Verification items for the finished model (mm, model axes). A direction names the side the tool comes from. Coordinates: 2 decimals unless noted, no trailing zeros. Write each loop counter-clockwise with the first axis right and the second up, starting at its lowest first coordinate (ties: lowest second). Pieces come first, ordered by that corner, then holes. Notation, with made-up numbers: M 18,44 L 56,44 A21 cw 56,83 Z; hole C 34,1.25 d5. An arc over 180 degrees is marked long. One line per item, written item: value.
```python
from build123d import *

# Parameters (mm, degrees)
SKETCH2_W           = 220
SKETCH2_H           = 140
BOSS_EXTRUDE1_DEPTH = 2
CUT_EXTRUDE1_DEPTH  = 2
SKETCH4_W           = 8
SKETCH4_H           = 20
BOSS_EXTRUDE2_DEPTH = 2
SKETCH5_W           = 4
SKETCH5_H           = 4.381248614
BOSS_EXTRUDE3_DEPTH = 20


with BuildPart() as part:
    # Sketch2 → Boss-Extrude1 (new body)
    with BuildSketch(Plane(origin=(0, 0, 0), x_dir=(1, 0, 0), z_dir=(0, 1, 0))):
        Rectangle(SKETCH2_W, SKETCH2_H)
    extrude(amount=BOSS_EXTRUDE1_DEPTH)

    # Sketch3 → Cut-Extrude1 (cut)
    with BuildSketch(Plane(origin=(0, 0, 0), x_dir=(1, 0, 0), z_dir=(0, 1, 0))):
        Polygon((-80, -35), (-80, -22), (-85, -22), (-85, -68), (-80, -68), (-80, -55), (80, -55), (80, -68), (85, -68), (85, -22), (80, -22), (80, -35), align=None)
    extrude(amount=CUT_EXTRUDE1_DEPTH, mode=Mode.SUBTRACT)

    # Sketch4 → Boss-Extrude2 (add)
    with BuildSketch(Plane(origin=(0, 0, 0), x_dir=(1, 0, 0), z_dir=(0, 1, 0))):
        with Locations((0, -45)):
            Rectangle(SKETCH4_W, SKETCH4_H)
    extrude(amount=BOSS_EXTRUDE2_DEPTH)

    # Sketch5 → Boss-Extrude3 (add)
    with BuildSketch(Plane(origin=(0, 2, 0), x_dir=(1, 0, 0), z_dir=(0, 1, 0))):
        with Locations((-2, -42.809375693)):
            Rectangle(SKETCH5_W, SKETCH5_H)
    extrude(amount=BOSS_EXTRUDE3_DEPTH)


solid = part.part
```
Item 1: Cross-section at C-C, the plane y = 15.5. Enter the section's corners in (x, z).
The answers:
outline: M -4,40.62 L 0,40.62 L 0,45 L -4,45 Z
Item 2: Go/stop test with flat-tipped pins: P1, Ø10, axis at x = -72, y = 6.5, coming from the -Z side; P2, Ø10, axis at x = 34.5, z = 46, coming from the -Y side; P3, Ø1.2, axis at x = -1, y = 9, coming from the -Z side; P4, Ø3, axis at x = -1.5, y = 12, coming from the +Z side. Record where each tip stops, or that it passes through.
The answers:
P1: stops at z = -70
P2: passes through
P3: stops at z = 40.62
P4: stops at z = 45
Item 3: Draft check along X on faces 1 (the face through (-2, 0, -1)), 2 (the face through (-4, 9, 44)), 3 (the face through (0, 12, 43)). Enter one of: released by +X, released by -X, zero draft, split by the parting line, or undercut.
The answers:
face 1: zero draft
face 2: undercut
face 3: released by +X
Item 4: Access from +Z, -Z, +X, -X, +Y, -Y to the whole of each face (thin tool, end or side, straight path). Record for faces 4 (the face through (-2, 12, 45)), 5 (the face through (-2, 22, 43)), 6 (the face through (-2, 12, 40.619)).
The answers:
face 4: +Z, +X, -X, +Y
face 5: +Z, -Z, +X, -X, +Y
face 6: -Z, +X, -X, +Y
Item 5: Cross-section at B-B, the plane x = -73. Enter the section's corners in (y, z).
The answers:
outline: M 0,-70 L 2,-70 L 2,35 L 0,35 Z; M 0,55 L 2,55 L 2,70 L 0,70 Z
Item 6: Scan line: line 1 (Y direction, x = 19.5, z = -31). Record every from-to range of solid material in increasing order.
The answers:
line 1: y = 0 to 2
Item 7: Cross-section at D-D, the plane z = -37. Enter the section's corners in (x, y), and give its area (3 significant figures).
The answers:
outline: M -110,0 L 110,0 L 110,2 L -110,2 Z
area: 440 mm²
Item 8: Cross-section at A-A, the plane z = 27. Enter the section's corners in (x, y).
The answers:
outline: M -110,0 L -85,0 L -85,2 L -110,2 Z; M -80,0 L 80,0 L 80,2 L -80,2 Z; M 85,0 L 110,0 L 110,2 L 85,2 Z
